For this review, take the finished solid that the model builds, in its own axes (mm). Face numbers are marked on the shaded views. A direction names the side the tool comes from. Coordinates: 2 decimals unless noted, no trailing zeros. Write each loop counter-clockwise with the first axis right and the second up, starting at its lowest first coordinate (ties: lowest second). Pieces come first, ordered by that corner, then holes. Notation, with made-up numbers: (79, 50.25) - (84, 50.25) arc R36 cw to (84, 87.25) - close; hole circle Ø9 at (58.25, 5). An arc over 180 degrees is marked (long way). Use one line per item in the form item = value. Start each with the question number.
1) Insertion check: P1, Ø5.5, axis at x = 25, y = 11.5, coming from the +Z side; P2, Ø8, axis at x = 7.5, y = 15, coming from the -Z side; P3, Ø1.6, axis at x = -3.5, y = -1, coming from the -Z side. Each pin has a flat end and moves straight along its axis. Give the tip position at first contact, or say it passes through.
2) Tool access review of the marked faces 1 and 2: name each direction out of +Z, -Z, +X, -X, +Y, -Y from which nothing blocks a thin tool from reaching the whole face with its end or side.
3) For L1, parallel to Z at x = 40, y = 2.75; L2, parallel to Y at x = 17.5, z = -4.25; L3, parallel to X at y = -0.95, z = 3, list the stretches that pass through material, from the lowest coordinate up. Write a range as from..to.
4) We need section B-B (x = 31). Give the boundary of the cut face in (y, z), plus the area to 3 significant figures.
5) We need section A-A (x = -4). Give the boundary of the cut face in (y, z).
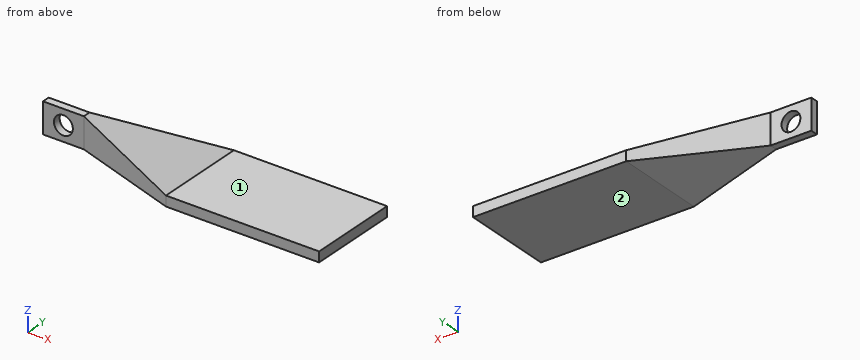
```python
from build123d import *

# Parameters (mm, degrees)
SKETCH_1_W          = 8
SKETCH_1_H          = 1.5
EXTRUDE_1_DEPTH     = 6
SKETCH_2_W          = 30
SKETCH_2_H          = 2
EXTRUDE_2_DEPTH     = 18
SKETCH_3_R          = 1.85
CUT_EXTRUDE_1_DEPTH = 6


with BuildPart() as part:
    # 草图1 → 凸台-拉伸1 (new body)
    with BuildSketch(Plane.XY):
        with Locations((-4, -0.75)):
            Rectangle(SKETCH_1_W, SKETCH_1_H)
    extrude(amount=EXTRUDE_1_DEPTH)


with BuildPart() as body_2:
    # 草图2 → 凸台-拉伸2 (new body)
    with BuildSketch(Plane(origin=(0, 0, 0), x_dir=(1, 0, 0), z_dir=(0, 1, 0))):
        with Locations((30, 5)):
            Rectangle(SKETCH_2_W, SKETCH_2_H)
    extrude(amount=EXTRUDE_2_DEPTH)


    add(part.part)  # loft_1 joins it to this body
    # loft from a face of the part (loft_1)
    loft([body_2.faces().sort_by_distance((15, 9, -5))[0], body_2.faces().sort_by_distance((0, -0.75, 3))[0]])

    # 草图3 → 切除-拉伸1 (cut)
    with BuildSketch(Plane(origin=(0, 0, 0), x_dir=(1, 0, 0), z_dir=(0, 1, 0))):
        with Locations(Location((-4, -3, 0), (0, 0, 270))):
            Circle(SKETCH_3_R)
    extrude(amount=-CUT_EXTRUDE_1_DEPTH, mode=Mode.SUBTRACT)


solid = body_2.part
```
Determined:
q1.P1 = -4
q1.P2 = -4.47
q1.P3 = 0
q2.face_1 = +Z, +X, +Y, -Y
q2.face_2 = -Z, +X, -X, +Y, -Y
q3.L1 = -6..-4
q3.L2 = 0..18
q3.L3 = -8..-5.85, -2.15..4.5
q4.outline = (0, -6) - (18, -6) - (18, -4) - (0, -4) - close
q4.area = 36.0 mm²
q5.outline = (-1.5, 0) - (0, 0) - (0, 1.15) - (-1.5, 1.15) - close; (-1.5, 4.85) - (0, 4.85) - (0, 6) - (-1.5, 6) - close
